Can you work these out from the model? Positions are in its coordinate system, mm. Round coordinates to 2 decimals unless told otherwise and drop trailing zeros. Order: outer loops, then holes, each group sorted by start corner. A loop starts at its lowest first (then second) coordinate and runs counter-clockwise, first axis right, second up. Notation, with made-up numbers: M -12.5,47 L 34.5,47 A23 ccw 34.5,74 Z; hole C -7,78 d9. An arc over 180 degrees is marked long. Answer as a JSON object with one key per item and string values. Group by question number.
```python
from build123d import *

# Parameters (mm, degrees)
SKETCH2_R           = 1.65
BOSS_EXTRUDE1_DEPTH = 6
CUT_EXTRUDE1_DEPTH  = 110.659974352


with BuildPart() as part:
    # Sketch2 → Boss-Extrude1 (new body)
    with BuildSketch(Plane.XY):
        with BuildLine():
            ThreePointArc((90, -18.005197753), (108.005197753, 0), (90, 18.005197753))
            add(Edge.make_bspline(
                [(90, 18.005197753), (87.300427685, 18.005389985), (81.17457593, 17.968478919), (73.674128402, 17.806885767), (68.874876564, 17.634447138), (67.5, 17.578928476)],
                knots=[0.344744853, 0.344744853, 0.344744853, 0.344744853, 0.357984483, 0.374788114, 0.381536428, 0.381536428, 0.381536428, 0.381536428], degree=3))
            ThreePointArc((67.5, 17.578928476), (85.803106629, 0), (67.5, -17.578928476))
            add(Edge.make_bspline(
                [(67.5, -17.578928476), (68.874876564, -17.634447138), (73.674128402, -17.806885767), (81.17457593, -17.968478919), (87.300427685, -18.005389985), (90, -18.005197753)],
                knots=[0.618463572, 0.618463572, 0.618463572, 0.618463572, 0.625211886, 0.642015517, 0.655255147, 0.655255147, 0.655255147, 0.655255147], degree=3))
        make_face()
        with Locations((90, 0)):
            Circle(SKETCH2_R, mode=Mode.SUBTRACT)
    extrude(amount=BOSS_EXTRUDE1_DEPTH)

    # Sketch3 → Cut-Extrude1 (cut, through all)
    with BuildSketch(Plane.XY.offset(6)):
        with BuildLine():
            Line((88.025921382, 18.002375731), (90, 17.705197753))
            ThreePointArc((90, 17.705197753), (107.705197753, 0), (90, -17.705197753))
            Line((90, -17.705197753), (88.025921382, -18.002375731))
            add(Edge.make_bspline(
                [(88.025921382, -18.002375731), (88.683945552, -18.004313587), (89.341972833, -18.00524461), (90, -18.005197753)],
                knots=[0.652027956, 0.652027956, 0.652027956, 0.652027956, 0.655255147, 0.655255147, 0.655255147, 0.655255147], degree=3))
            ThreePointArc((90, -18.005197753), (108.005197753, 0), (90, 18.005197753))
            add(Edge.make_bspline(
                [(90, 18.005197753), (89.341972833, 18.00524461), (88.683945552, 18.004313587), (88.025921382, 18.002375731)],
                knots=[0.344744853, 0.344744853, 0.344744853, 0.344744853, 0.347972044, 0.347972044, 0.347972044, 0.347972044], degree=3))
        make_face()
    extrude(amount=-CUT_EXTRUDE1_DEPTH, mode=Mode.SUBTRACT)


solid = part.part
```
1) We'd pull the mould along X, two halves only. Please class faces 1 (the face through (88.35, 0.07, 2.96)), 2 (the face through (92, 0, 6)), 3 (the face through (107.7, 0.4, 3)): +X half, -X half, draft (parallel to the pull), parting line (faces both ways), or undercut.
2) If we section it at B-B on x = 103: Write out the boundary of the cut face in (y, z), plus the area to 3 significant figures.
3) For pin 1 (10 mm diameter, centred on x = 98.5, y = 14, fed in from -Z); pin 2 (3 mm diameter, centred on y = 4.5, z = 2, fed in from -X); pin 3 (3 mm diameter, centred on y = 3, z = 4.5, fed in from -X); pin 4 (2 mm diameter, centred on y = 0, z = 4.5, fed in from -X), each with a flat end and sliding along its axis, tell me the tip position at first contact or that it passes through.
4) If we section it at A-A on y = 0: Write out the boundary of the cut face in (x, z), plus the area to 3 significant figures.
5) I need wall thicknesses on line 1 along Y through (x, z) = (90, 1.5); line 2 along X through (y, z) = (1, 0.75); line 3 along Y through (x, z) = (80, 3.5). Which ranges of each line are inside material? Lowest first, please.
Findings:
{
 "1": {"face 1": "undercut", "face 2": "draft", "face 3": "+X half"},
 "2": {"outline": "M -12.02,0 L 12.02,0 L 12.02,6 L -12.02,6 Z", "area": "144 mm^2"},
 "3": {"pin 1": "stops at z = 0", "pin 2": "stops at x = 84.75", "pin 3": "stops at x = 85.22", "pin 4": "stops at x = 85.77"},
 "4": {"outline": "M 85.8,0 L 88.35,0 L 88.35,6 L 85.8,6 Z; M 91.65,0 L 107.71,0 L 107.71,6 L 91.65,6 Z", "area": "112 mm^2"},
 "5": {"line 1": "y = -17.71 to -1.65, 1.65 to 17.71", "line 2": "x = 85.77 to 88.69, 91.31 to 107.68", "line 3": "y = -17.93 to -13.06, 13.06 to 17.93"}
}
